```python
from build123d import *

# Parameters (mm, degrees)
F0_W     = 694
F0_H     = 218
F1_DEPTH = 18
F2_R     = 12.5
F3_DEPTH = 4


with BuildPart() as f1:
    # F0 (on Front) → F1 (new body)
    with BuildSketch(Plane.XZ):
        Rectangle(F0_W, F0_H)
    extrude(amount=F1_DEPTH)

    # F2 (on face) → F3 (join)
    with BuildSketch(Plane.XZ.offset(18)):
        with Locations((0, 70)):
            Circle(F2_R)
    extrude(amount=F3_DEPTH)


solid = f1.part
```
Work out the finished part from the listing and answer in its coordinate system (mm). A direction names the side the tool comes from. Round coordinates to 2 decimals unless told otherwise and drop trailing zeros. Write each loop counter-clockwise with the first axis right and the second up, starting at its lowest first coordinate (ties: lowest second). Pieces come first, ordered by that corner, then holes. Notation, with made-up numbers: (-0.75, 80.25) -> (37.25, 80.25) arc R35 cw to (37.25, 118.25) -> close; hole circle Ø4 at (-35.75, -27). An arc over 180 degrees is marked (long way). Write each question's results on one line, items separated by ' | '.
1) Flat-ended cylindrical pins translate along their axes: pin 1 (3 mm diameter, centred on x = -20.5, z = -85, fed in from -Y); pin 2 (3 mm diameter, centred on x = -252.5, z = -48.5, fed in from +Y). Find the tip coordinate at first contact, or state that the pin passes through.
Findings:
pin 1: stops at y = -18 | pin 2: stops at y = 0
2) The part is cut by section B-B (z = 70). Write down the section's boundary in (x, y).
Findings:
outline: (-347, -18) -> (-12.5, -18) -> (-12.5, -22) -> (12.5, -22) -> (12.5, -18) -> (347, -18) -> (347, 0) -> (-347, 0) -> close
3) The part is cut by section C-C (x = 239). Write down the section's boundary in (y, z).
Findings:
outline: (-18, -109) -> (0, -109) -> (0, 109) -> (-18, 109) -> close
4) Which of the six approach directions +Z, -Z, +X, -X, +Y, -Y give full straight-line access (tool end or side, diameter ignored) to faces 1 (the cylindrical face through (-1.627, -19.972, 82.394)), 2 (the flat face through (-347, -9, -2))?
Findings:
face 1: -Y | face 2: +Z, -Z, -X, +Y, -Y
5) Consider line 1 along Y through (x, z) = (274, 2.5). Determine where the line is inside the solid, lowest interval first. Write a range as [from, to].
Findings:
line 1: y = [-18, 0]
6) The part is cut by section A-A (x = 0). Write down the section's boundary in (y, z).
Findings:
outline: (-22, 57.5) -> (-18, 57.5) -> (-18, -109) -> (0, -109) -> (0, 109) -> (-18, 109) -> (-18, 82.5) -> (-22, 82.5) -> close
